```python
from build123d import *

# Parameters (mm, degrees)
SKETCH_1_W          = 96
SKETCH_1_H          = 70
EXTRUDE_1_DEPTH     = 10
FILLET_1_R          = 10
SKETCH_2_R          = 2.6
CUT_EXTRUDE_1_DEPTH = 10
SKETCH_3_R          = 5
CUT_EXTRUDE_2_DEPTH = 5
SKETCH_4_R          = 3.1
CUT_EXTRUDE_3_DEPTH = 5
CHAMFER_1_SIZE      = 1
CHAMFER_2_SIZE      = 2
SKETCH_5_W          = 50
SKETCH_5_H          = 30
CUT_EXTRUDE_4_DEPTH = 10
FILLET_2_R          = 10
CHAMFER_3_SIZE      = 2


with BuildPart() as part:
    # 草图1 → 凸台-拉伸1 (new body)
    with BuildSketch(Plane.XY):
        Rectangle(SKETCH_1_W, SKETCH_1_H)
    extrude(amount=EXTRUDE_1_DEPTH)

    # 圆角1
    fillet_1_edges = [part.edges().sort_by_distance(p)[0] for p in [
        (48, -35, 5),
        (-48, -35, 5),
        (-48, 35, 5),
        (48, 35, 5),
    ]]
    fillet(fillet_1_edges, radius=FILLET_1_R)

    # 草图2 → 切除-拉伸1 (cut)
    with BuildSketch(Plane.XY.offset(10)):
        with Locations((0, 25.5)):
            Circle(SKETCH_2_R)
        with Locations((-12.7, 25.5)):
            Circle(SKETCH_2_R)
        with Locations((12.7, 25.5)):
            Circle(SKETCH_2_R)
        with Locations((-12.7, -25.5)):
            Circle(SKETCH_2_R)
        with Locations((0, -25.5)):
            Circle(SKETCH_2_R)
        with Locations((12.7, -25.5)):
            Circle(SKETCH_2_R)
    extrude(amount=-CUT_EXTRUDE_1_DEPTH, mode=Mode.SUBTRACT)

    # 草图3 → 切除-拉伸2 (cut)
    with BuildSketch(Plane.XY.offset(10)):
        with Locations((-38, 25)):
            Circle(SKETCH_3_R)
        with Locations((-38, 0)):
            Circle(SKETCH_3_R)
        with Locations((-38, -25)):
            Circle(SKETCH_3_R)
        with Locations((38, -25)):
            Circle(SKETCH_3_R)
        with Locations((38, 0)):
            Circle(SKETCH_3_R)
        with Locations((38, 25)):
            Circle(SKETCH_3_R)
    extrude(amount=-CUT_EXTRUDE_2_DEPTH, mode=Mode.SUBTRACT)

    # 草图4 → 切除-拉伸3 (cut)
    with BuildSketch(Plane.XY.offset(5)):
        with Locations((-38, 25)):
            Circle(SKETCH_4_R)
        with Locations((-38, 0)):
            Circle(SKETCH_4_R)
        with Locations((-38, -25)):
            Circle(SKETCH_4_R)
        with Locations((38, 25)):
            Circle(SKETCH_4_R)
        with Locations((38, 0)):
            Circle(SKETCH_4_R)
        with Locations((38, -25)):
            Circle(SKETCH_4_R)
    extrude(amount=-CUT_EXTRUDE_3_DEPTH, mode=Mode.SUBTRACT)

    # 倒角1
    chamfer_1_edges = [part.edges().sort_by_distance(p)[0] for p in [
        (34.9, 0, 0),
        (34.9, -25, 0),
        (-41.1, 25, 0),
        (-41.1, 0, 0),
        (-41.1, -25, 0),
        (34.9, 25, 0),
    ]]
    chamfer(chamfer_1_edges, length=CHAMFER_1_SIZE)

    # 倒角2
    chamfer_2_edges = [part.edges().sort_by_distance(p)[0] for p in [
        (0, 35, 10),
        (48, 0, 10),
        (-48, 0, 10),
        (0, -35, 10),
        (-45.071067812, -32.071067812, 10),
        (45.071067812, -32.071067812, 10),
        (-45.071067812, 32.071067812, 10),
        (45.071067812, 32.071067812, 10),
    ]]
    chamfer(chamfer_2_edges, length=CHAMFER_2_SIZE)

    # 草图5 → 切除-拉伸4 (cut)
    with BuildSketch(Plane.XY.offset(10)):
        Rectangle(SKETCH_5_W, SKETCH_5_H)
    extrude(amount=-CUT_EXTRUDE_4_DEPTH, mode=Mode.SUBTRACT)

    # 圆角2
    fillet_2_edges = [part.edges().sort_by_distance(p)[0] for p in [
        (25, 15, 5),
        (25, -15, 5),
        (-25, -15, 5),
        (-25, 15, 5),
    ]]
    fillet(fillet_2_edges, radius=FILLET_2_R)

    # 倒角3
    chamfer_3_edges = [part.edges().sort_by_distance(p)[0] for p in [
        (25, 0, 10),
        (25, 0, 0),
        (0, -15, 10),
        (0, -15, 0),
        (0, 15, 10),
        (0, 15, 0),
        (-25, 0, 10),
        (-25, 0, 0),
        (22.071067812, -12.071067812, 10),
        (22.071067812, -12.071067812, 0),
        (22.071067812, 12.071067812, 10),
        (22.071067812, 12.071067812, 0),
        (-22.071067812, -12.071067812, 10),
        (-22.071067812, -12.071067812, 0),
        (-22.071067812, 12.071067812, 10),
        (-22.071067812, 12.071067812, 0),
    ]]
    chamfer(chamfer_3_edges, length=CHAMFER_3_SIZE)


solid = part.part
```
Read the model definition and answer for the solid it produces. Units are mm, in the model's axes. A direction names the side the tool comes from. Give positions to 0.01 mm unless a question says otherwise; leave off trailing zeros. Loops run counter-clockwise (first coordinate to the right, second up) from the corner with the lowest first, then second, coordinate; pieces in that order, holes last.
Item 1: Find the intervals of material crossed by line 1 along Y through (x, z) = (-12.5, 7.25); line 2 along Y through (x, z) = (-38, 2.5); line 3 along X through (y, z) = (5.5, 8), in increasing order.
Item 2: For faces 4 (the cylindrical face through (33, 0, 8)), 5 (the flat face through (0, 15, 5)), 6 (the conical face through (-22.536, -12.372, 1.458)), determine the directions among +Z, -Z, +X, -X, +Y, -Y from which every point of the face is accessible in a straight line to the end or side of a thin tool.
Item 3: Each of these flat-tipped pins is pushed along its axis until it touches: pin 1 Ø5 at (x, y) = (17, 10.5) entering from +Z (3 decimals); pin 2 Ø1 at (x, y) = (18.5, 15.5) entering from -Z; pin 3 Ø8 at (x, y) = (-38, 0) entering from -Z; pin 4 Ø8 at (x, y) = (38, 0) entering from +Z. Where does it stop, or does it pass through?
Item 4: The part is cut by section A-A (x = 0). Write down the section's boundary in (y, z), and give its area (3 significant figures).
Item 5: The mould has two halves that part along X. Classify faces 1 (the flat face through (47, 0, 9)), 2 (the cylindrical face through (-43, 0, 8)), 3 (the conical face through (22.536, 12.372, 1.458)): released by +X, released by -X, zero draft, split by the parting line, or undercut.
Item 6: The part is cut by section B-B (z = 4). Give the number of separate pieces and of enclosed holes in the cut face, and give its area (3 significant figures).
Taken from the geometry:
1. line 1: y = -35 to -28.09, -22.91 to -15, 15 to 22.91, 28.09 to 35
1. line 2: y = -35 to -28.1, -21.9 to -3.1, 3.1 to 21.9, 28.1 to 35
1. line 3: x = -48 to -24.99, 24.99 to 48
2. face 4: +Z
2. face 5: +Z, -Z
2. face 6: -Z
3. pin 1: passes through
3. pin 2: stops at z = 0.43
3. pin 3: stops at z = 0.1
3. pin 4: stops at z = 5
4. outline: (-35, 0) - (-28.1, 0) - (-28.1, 10) - (-33, 10) - (-35, 8) - close; (-22.9, 0) - (-17, 0) - (-15, 2) - (-15, 8) - (-17, 10) - (-22.9, 10) - close; (15, 2) - (17, 0) - (22.9, 0) - (22.9, 10) - (17, 10) - (15, 8) - close; (28.1, 0) - (35, 0) - (35, 8) - (33, 10) - (28.1, 10) - close
4. area: 284 mm2
5. face 1: released by +X
5. face 2: undercut
5. face 3: undercut
6. separate pieces: 1
6. enclosed holes: 13
6. area: 4,910 mm2
